The model under review builds one solid part; all positions refer to its coordinate system, in mm. Round coordinates to 2 decimals unless told otherwise and drop trailing zeros. Write each loop counter-clockwise with the first axis right and the second up, starting at its lowest first coordinate (ties: lowest second). Pieces come first, ordered by that corner, then holes. Notation, with made-up numbers: (63.25, 59.25) -> (95.25, 59.25) arc R25 cw to (95.25, 88.25) -> close; hole circle Ø7 at (22.25, -23.5). An arc over 180 degrees is marked (long way). Answer as a JSON object with one key per item and string values. Group by question number.
1) We need section B-B, the plane z = 7.5. Write out the cut boundary in (x, y), then the cut area to 3 significant figures.
2) We need section A-A, the plane y = 0. Write out the cut boundary in (x, z), then the cut area to 3 significant figures.
3) To check wall thickness, follow probe 1 along Y at (x, z) = (6, 7.5); probe 2 along Y at (x, z) = (12, 5.75); probe 3 along X at (y, z) = (2, 6). State the ranges of each line that lie inside material, in increasing order. Write a range as [from, to].
4) Insertion check: pin 1 Ø5 at (y, z) = (29.5, 7.5) entering from +X; pin 2 Ø5 at (x, z) = (21.5, 5) entering from +Y; pin 3 Ø2 at (x, z) = (25, 5) entering from -Y; pin 4 Ø5 at (x, y) = (-20, 7.5) entering from +Z. Each pin has a flat end and moves straight along its axis. Give the tip position at first contact, or say it passes through.
5) Mouldability with a two-part tool opening along Y and no side actions: class faces 1 (the cylindrical face through (-20.633, -15.821, 7.395)), 2 (the flat face through (15, -22, 15)), 3 (the cylindrical face through (-24.322, 22.303, 7.395)) as pulls with the +Y half, pulls with the -Y half, needs draft (parallel to the pull), parting line crosses it, or undercut.
6) We need section C-C, the plane x = -7. Write out the cut boundary in (y, z).
7) We need section D-D, the plane x = -22. Write out the cut boundary in (y, z).
from build123d import *

# Parameters (mm, degrees)
F0_R          = 33
F0_R_2        = 26
F1_DEPTH      = 15
F2_R          = 2
F3_DEPTH      = 33.001
F3_DEPTH_BACK = 33.001


with BuildPart() as f1:
    # F0 (on Top) → F1 (new body)
    with BuildSketch(Plane.XY):
        Circle(F0_R)
        Circle(F0_R_2, mode=Mode.SUBTRACT)
    extrude(amount=F1_DEPTH)

    # F2 (on Right) → F3 (cut, two sides)
    with BuildSketch(Plane.YZ) as f3_sk:
        with Locations((29.5, 7.5)):
            Circle(F2_R)
        with Locations((-29.5, 7.5)):
            Circle(F2_R)
    extrude(amount=-F3_DEPTH, mode=Mode.SUBTRACT)
    extrude(f3_sk.sketch, amount=F3_DEPTH_BACK, mode=Mode.SUBTRACT)


solid = f1.part
Here are the results:
{
 "1": {"outline": "(-18.24, -27.5) -> (18.24, -27.5) arc R33 ccw to (18.24, 27.5) -> (-18.24, 27.5) arc R33 ccw to start; (-9.84, -31.5) arc R33 ccw to (9.84, -31.5) -> close; (-9.84, 31.5) -> (9.84, 31.5) arc R33 ccw to start; hole circle Ø52 at (0, 0)", "area": "1,060 mm^2"},
 "2": {"outline": "(-33, 0) -> (-26, 0) -> (-26, 15) -> (-33, 15) -> close; (26, 0) -> (33, 0) -> (33, 15) -> (26, 15) -> close", "area": "210 mm^2"},
 "3": {"probe 1": "y = [-32.45, -31.5], [-27.5, -25.3], [25.3, 27.5], [31.5, 32.45]", "probe 2": "y = [-30.74, -30.47], [-28.53, -23.07], [23.07, 28.53], [30.47, 30.74]", "probe 3": "x = [-32.94, -25.92], [25.92, 32.94]"},
 "4": {"pin 1": "stops at x = 18.97", "pin 2": "stops at y = 26.98", "pin 3": "stops at y = -22.65", "pin 4": "passes through"},
 "5": {"face 1": "undercut", "face 2": "needs draft", "face 3": "parting line crosses it"},
 "6": {"outline": "(-32.25, 0) -> (-25.04, 0) -> (-25.04, 15) -> (-32.25, 15) -> close; (25.04, 0) -> (32.25, 0) -> (32.25, 15) -> (25.04, 15) -> close; hole circle Ø4 at (-29.5, 7.5); hole circle Ø4 at (29.5, 7.5)"},
 "7": {"outline": "(-24.6, 0) -> (-13.86, 0) -> (-13.86, 15) -> (-24.6, 15) -> close; (13.86, 0) -> (24.6, 0) -> (24.6, 15) -> (13.86, 15) -> close"}
}
